Input: dimensioned drawing with shaded views. Units: mm. Origin: part minimum x, y, z. A direction names the side the tool comes from. Give positions to 0.01 mm unless a question says otherwise; leave off trailing zeros. Loops run counter-clockwise (first coordinate to the right, second up) from the corner with the lowest first, then second, coordinate; pieces in that order, holes last. Notation, with made-up numbers: (50, 79.5) -> (61, 79.5) arc R30 ccw to (61, 111.5) -> close; hole circle Ø10 at (10, -26). An arc over 180 degrees is marked (long way). One line per question, with ' | ' between items. Start each with the question number.
Item 1: Material intervals for line 1 along Y through (x, z) = (6.5, 1.5) (3 decimals); line 2 along Y through (x, z) = (14.5, 8.5) (3 decimals); line 3 along Z through (x, y) = (19.75, 24), sorted ascending. Write a range as [from, to].
Item 2: Section C-C on y = 16.75. Return loops of the section in (x, z) (1 decimal).
Item 3: Section B-B on z = 11.5. Return loops of the section in (x, y) (3 decimals), then the cut area to 3 significant figures.
Item 4: Set-up query: the marked faces 1 and 2. Return all of +Z, -Z, +X, -X, +Y, -Y with unobstructed straight access to the full face (end or side cutting, diameter ignored); none if empty.
Item 5: Section D-D on x = 14.5. Return loops of the section in (y, z) (3 decimals), then the cut area to 3 significant figures.
Item 6: Section A-A on x = 11.25. Return loops of the section in (y, z) (3 decimals).
Item 7: Pin query (flat end, axial travel): P1, Ø1.5, axis at x = 3.5, z = 12.5, coming from the -Y side (3 decimals); P2, Ø6, axis at y = 13, z = 18, coming from the +X side; P3, Ø10, axis at x = 5.5, y = 24, coming from the -Z side. Return the tip coordinate at first contact, or that it passes through.
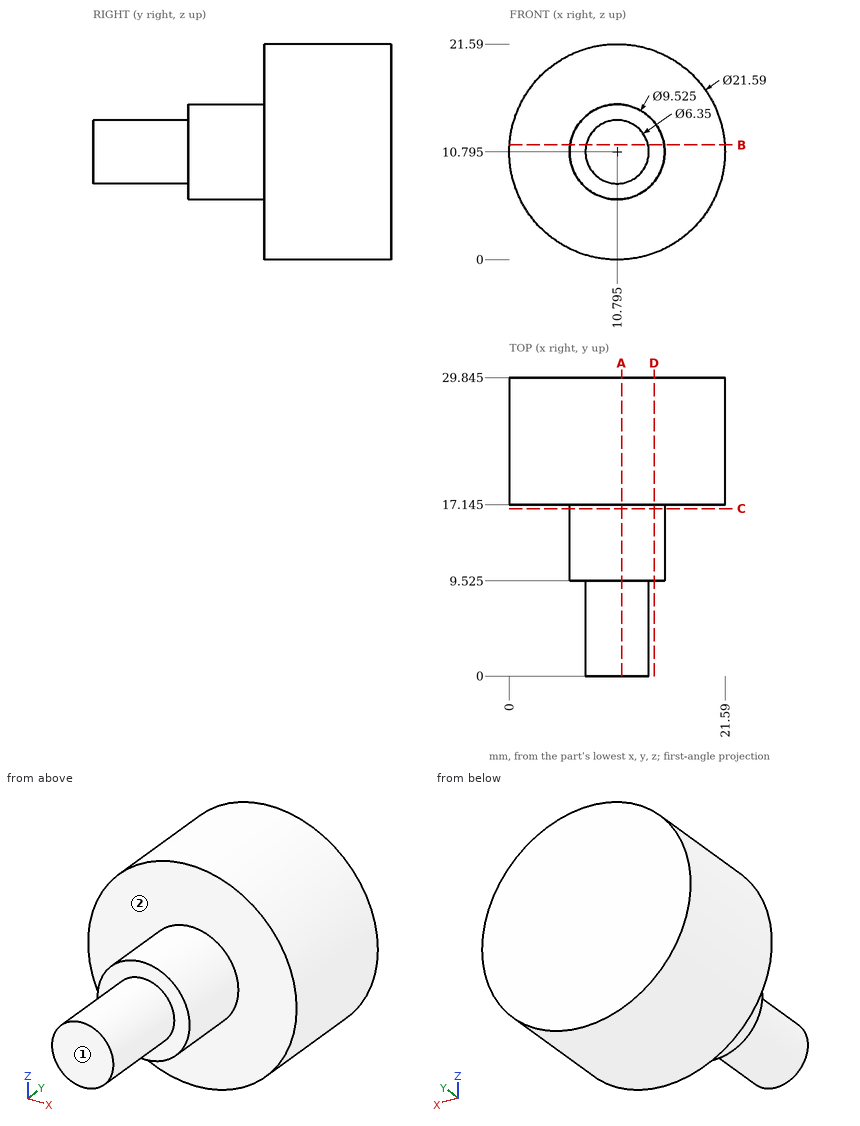
Result sheet:
1) line 1: y = [17.145, 29.845] | line 2: y = [9.525, 29.845] | line 3: z = [4.77, 16.82]
2) outline: circle Ø9.5 at (10.8, 10.8)
3) outline: (0.023, 17.145) -> (6.085, 17.145) -> (6.085, 9.525) -> (7.699, 9.525) -> (7.699, 0) -> (13.891, 0) -> (13.891, 9.525) -> (15.505, 9.525) -> (15.505, 17.145) -> (21.567, 17.145) -> (21.567, 29.845) -> (0.023, 29.845) -> close | area: 404 mm²
4) face 1: +Z, -Z, +X, -X, -Y | face 2: -Y
5) outline: (9.525, 7.803) -> (17.145, 7.803) -> (17.145, 0.656) -> (29.845, 0.656) -> (29.845, 20.934) -> (17.145, 20.934) -> (17.145, 13.787) -> (9.525, 13.787) -> close | area: 303 mm²
6) outline: (0, 7.653) -> (9.525, 7.653) -> (9.525, 6.054) -> (17.145, 6.054) -> (17.145, 0.01) -> (29.845, 0.01) -> (29.845, 21.58) -> (17.145, 21.58) -> (17.145, 15.536) -> (9.525, 15.536) -> (9.525, 13.937) -> (0, 13.937) -> close
7) P1: stops at y = 17.145 | P2: stops at x = 13.03 | P3: stops at z = 0
